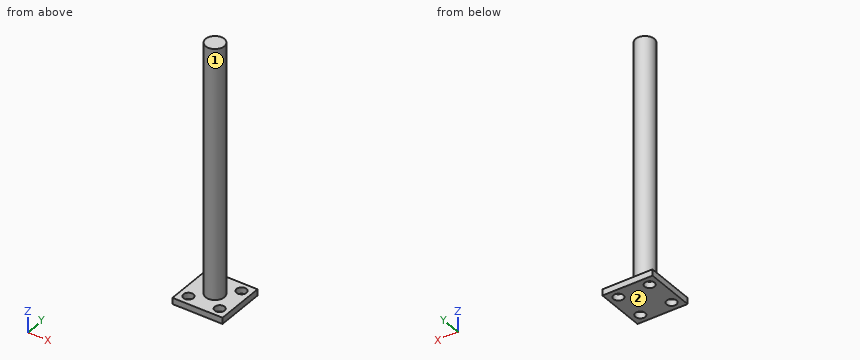
```python
from build123d import *

# Parameters (mm, degrees)
SKETCH_1_W      = 40
SKETCH_1_H      = 40
SKETCH_1_R      = 4
EXTRUDE_1_DEPTH = 5
SKETCH_2_R      = 7.5
EXTRUDE_2_DEPTH = 200


with BuildPart() as part:
    # 草图1 → 凸台-拉伸1 (new body)
    with BuildSketch(Plane.XY):
        Rectangle(SKETCH_1_W, SKETCH_1_H)
        with Locations((-12.5, 12.5)):
            Circle(SKETCH_1_R, mode=Mode.SUBTRACT)
        with Locations((12.5, 12.5)):
            Circle(SKETCH_1_R, mode=Mode.SUBTRACT)
        with Locations((12.5, -12.5)):
            Circle(SKETCH_1_R, mode=Mode.SUBTRACT)
        with Locations((-12.5, -12.5)):
            Circle(SKETCH_1_R, mode=Mode.SUBTRACT)
    extrude(amount=EXTRUDE_1_DEPTH)

    # 草图2 → 凸台-拉伸2 (add)
    with BuildSketch(Plane.XY.offset(5)):
        Circle(SKETCH_2_R)
    extrude(amount=EXTRUDE_2_DEPTH)


solid = part.part
```
For this review, take the finished solid that the model builds, in its own axes (mm). Face numbers are marked on the shaded views. A direction names the side the tool comes from. Give positions to 0.01 mm unless a question says otherwise; leave off trailing zeros. Write each loop counter-clockwise with the first axis right and the second up, starting at its lowest first coordinate (ties: lowest second). Pieces come first, ordered by that corner, then holes. Notation, with made-up numbers: M 84.25,25 L 139.25,25 A26 cw 139.25,62 Z; hole C 72,-22.75 d6. An arc over 180 degrees is marked long. Answer as a JSON object with one key per item and string values. Group by question number.
Item 1: Consider section B-B on x = 13.5. Write out the cut boundary in (y, z), plus the area to 3 significant figures.
Item 2: For probe 1 along Y at (x, z) = (12.5, 2.05); probe 2 along X at (y, z) = (-12, 1); probe 3 along Z at (x, y) = (1, -15), list the stretches that pass through material, from the lowest coordinate up. Write a range as [from, to].
Item 3: Tool access review of the marked faces 1 and 2: name each direction out of +Z, -Z, +X, -X, +Y, -Y from which nothing blocks a thin tool from reaching the whole face with its end or side.
Item 4: Consider section C-C on y = 0. Write out the cut boundary in (x, z), plus the area to 3 significant figures.
Item 5: For pin 1 Ø3 at (y, z) = (5, 129) entering from -X; pin 2 Ø10 at (y, z) = (-11.5, 35.5) entering from -X; pin 3 Ø10.5 at (x, y) = (-12.5, -12.5) entering from +Z, all flat-tipped, find the tip position at first contact; note any pin that passes through.
Item 6: Consider section A-A on y = 12.5. Write out the cut boundary in (x, z).
Item 7: Consider section D-D on z = 165. Write out the cut boundary in (x, y).
Check result:
{
 "1": {"outline": "M -20,0 L -16.37,0 L -16.37,5 L -20,5 Z; M -8.63,0 L 8.63,0 L 8.63,5 L -8.63,5 Z; M 16.37,0 L 20,0 L 20,5 L 16.37,5 Z", "area": "123 mm^2"},
 "2": {"probe 1": "y = [-20, -16.5], [-8.5, 8.5], [16.5, 20]", "probe 2": "x = [-20, -16.47], [-8.53, 8.53], [16.47, 20]", "probe 3": "z = [0, 5]"},
 "3": {"face 1": "+Z", "face 2": "-Z, +X, -X, +Y, -Y"},
 "4": {"outline": "M -20,0 L 20,0 L 20,5 L 7.5,5 L 7.5,205 L -7.5,205 L -7.5,5 L -20,5 Z", "area": "3,200 mm^2"},
 "5": {"pin 1": "stops at x = -6.63", "pin 2": "stops at x = -3.74", "pin 3": "stops at z = 5"},
 "6": {"outline": "M -20,0 L -16.5,0 L -16.5,5 L -20,5 Z; M -8.5,0 L 8.5,0 L 8.5,5 L -8.5,5 Z; M 16.5,0 L 20,0 L 20,5 L 16.5,5 Z"},
 "7": {"outline": "C 0,0 d15"}
}
